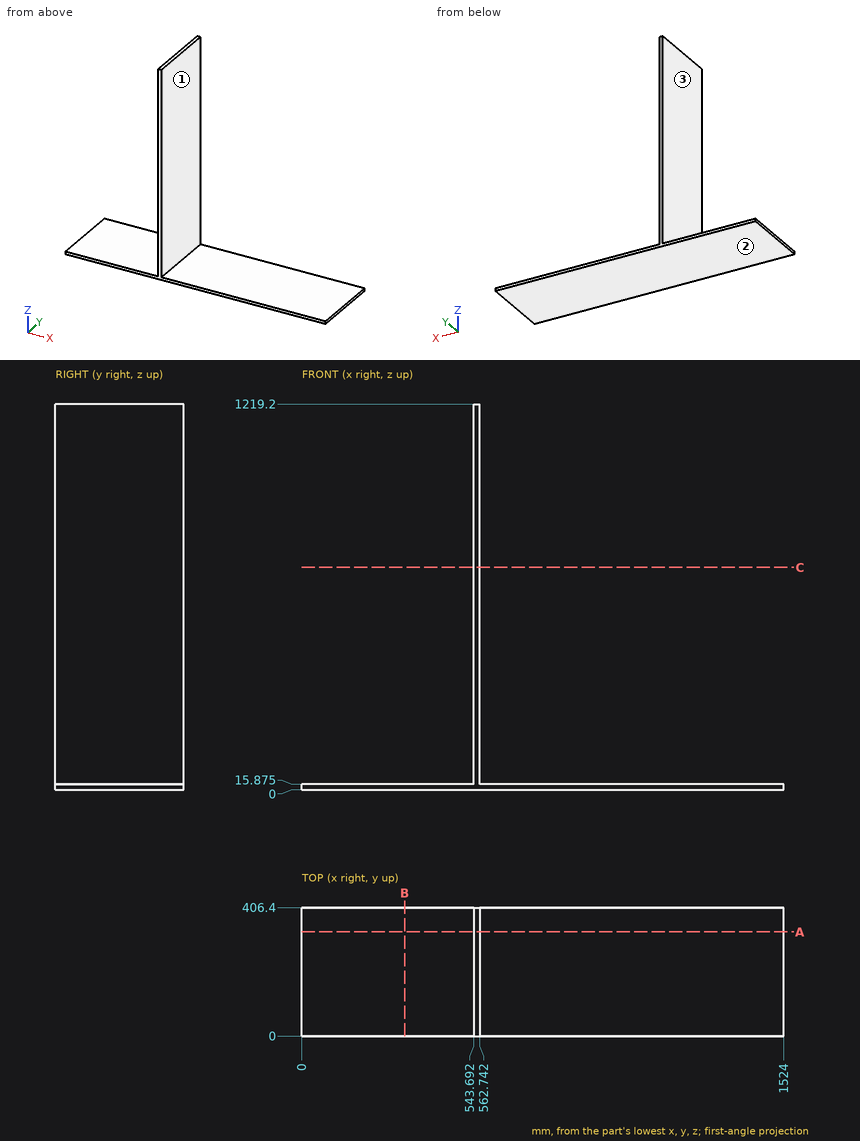
Can you work these out from the drawing? Everything is in mm from the part's minimum corner. A direction names the side the tool comes from. Give positions to 0.01 mm unless a question says otherwise; leave off trailing zeros. Loops run counter-clockwise (first coordinate to the right, second up) from the corner with the lowest first, then second, coordinate; pieces in that order, holes last. Notation, with made-up numbers: (-4.75, 62) -> (22.25, 62) arc R23 ccw to (22.25, 76) -> close; hole circle Ø8 at (-33.5, 31). An arc over 180 degrees is marked (long way). Return JSON: item names as keys, results as strings.
Item 1: If we section it at B-B on x = 325: List the corners of the cut face in (y, z) for me (3 decimals).
Geometry results:
{"outline": "(0, 0) -> (406.4, 0) -> (406.4, 15.875) -> (0, 15.875) -> close"}
Item 2: I need wall thicknesses on L1, parallel to X at y = 66.5, z = 905; L2, parallel to Z at x = 1234.5, y = 354 (3 decimals). Which ranges of each line are inside material? Lowest first, please. Write a range as from..to.
Geometry results:
{"L1": "x = 543.69..562.74", "L2": "z = 0..15.875"}
Item 3: If we section it at C-C on z = 702.5: List the corners of the cut face in (x, y) for me.
Geometry results:
{"outline": "(543.69, 0) -> (562.74, 0) -> (562.74, 406.4) -> (543.69, 406.4) -> close"}
Item 4: If we section it at A-A on y = 329: List the corners of the cut face in (x, z) for me (3 decimals).
Geometry results:
{"outline": "(0, 0) -> (1524, 0) -> (1524, 15.875) -> (562.742, 15.875) -> (562.742, 1219.2) -> (543.692, 1219.2) -> (543.692, 15.875) -> (0, 15.875) -> close"}
Item 5: I'm going to push flat-ended pins straight in: pin 1 (12 mm diameter, centred on y = 63.5, z = 809, fed in from -X); pin 2 (6 mm diameter, centred on x = 529.5, y = 196, fed in from +Z) (3 decimals). Where does each tip first touch, or does it pass through?
Geometry results:
{"pin 1": "stops at x = 543.69", "pin 2": "stops at z = 15.875"}
Item 6: Which directions (+Z, -Z, +X, -X, +Y, -Y) give clear straight access to the entire face, cutting with the end or side of a thin tool? Please do the marked faces 1, 2 and 3.
Geometry results:
{"face 1": "+Z, +X, +Y, -Y", "face 2": "-Z, +X, -X, +Y, -Y", "face 3": "+Z, -X, +Y, -Y"}
